Verification items for the finished model (mm, model axes). A direction names the side the tool comes from. Round coordinates to 2 decimals unless told otherwise and drop trailing zeros. Write each loop counter-clockwise with the first axis right and the second up, starting at its lowest first coordinate (ties: lowest second). Pieces come first, ordered by that corner, then holes. Notation, with made-up numbers: (-38.5, 1.25) - (-7.5, 1.25) arc R21 ccw to (-7.5, 5.25) - close; hole circle Ø6 at (27, 87). An arc over 180 degrees is marked (long way). Answer as a JSON object with one key per item and string values. Group by question number.
1) Mould release check, pull along Y, two halves, no side actions. Record for faces 5 (the cylindrical face through (-34.26, 7.31, 3.45)), 6 (the cylindrical face through (0, -15, 3)), 7 (the cylindrical face through (-14.287, -4.571, 3.451)), 8 (the cylindrical face through (39.73, 12.66, 3.45)): +Y half, -Y half, draft (parallel to the pull), parting line (faces both ways), or undercut.
2) Section check C-C (z = 6). Enter the section's corners in (x, y), then the cut area to 3 significant figures.
3) Section check B-B (y = -23.5). Enter the section's corners in (x, z), then the cut area to 3 significant figures.
4) Section check A-A (x = 0). Enter the section's corners in (y, z).
5) Go/stop test with flat-tipped pins: pin 1 Ø6 at (x, y) = (-7.5, -4.5) entering from +Z; pin 2 Ø1.5 at (x, z) = (-18, 6.5) entering from +Y; pin 3 Ø1 at (x, z) = (-6.5, 2.5) entering from +Y; pin 4 Ø2 at (y, z) = (18, 2) entering from +X. Record where each tip stops, or that it passes through.
6) Thickness scan on line 1 (Y direction, x = 17.5, z = 4.5); line 2 (X direction, y = -0.5, z = 6.5); line 3 (X direction, y = 17, z = 3). Record the ranges inside material, lowest first.
7) Set-up check for faces 1 (the flat face through (22.135, 2.461, 3.451)), 2 (the cylindrical face through (14.245, -4.7, 3.451)), 3 (the flat face through (-16.46, -15, 3.45)), 4 (the flat face through (19.6, 11.1, 3.5)): record each of +Z, -Z, +X, -X, +Y, -Y from which the full face is reachable in a straight line by a thin tool's end or side.
8) Section check D-D (y = 26). Enter the section's corners in (x, z).
```python
from build123d import *

# Parameters (mm, degrees)
F2_DEPTH = 7
F0_R     = 11.1
F3_DEPTH = 7.001
F4_R     = 3.652579
F5_DEPTH = 7.001


with BuildPart() as f2:
    # F1 (on Top) → F2 (new body)
    with BuildSketch(Plane.XY):
        with BuildLine():
            Line((-4.5, 29.528995), (-4.5, 14.309088))
            ThreePointArc((-4.5, 14.309088), (-8.816779, 12.135255), (-12.218175, 8.701506))
            Line((-12.218175, 8.701506), (-26.693166, 13.404716))
            ThreePointArc((-26.693166, 13.404716), (-39.661387, 12.886766), (-29.474319, 4.845207))
            Line((-29.474319, 4.845207), (-14.999328, 0.141997))
            ThreePointArc((-14.999328, 0.141997), (-14.265848, -4.635255), (-12.051247, -8.931262))
            Line((-12.051247, -8.931262), (-20.997284, -21.244425))
            ThreePointArc((-20.997284, -21.244425), (-24.512085, -33.737991), (-13.716131, -26.534492))
            Line((-13.716131, -26.534492), (-4.770094, -14.221329))
            ThreePointArc((-4.770094, -14.221329), (0, -15), (4.770094, -14.221329))
            Line((4.770094, -14.221329), (13.716131, -26.534492))
            ThreePointArc((13.716131, -26.534492), (24.512085, -33.737991), (20.997284, -21.244425))
            Line((20.997284, -21.244425), (12.051247, -8.931262))
            ThreePointArc((12.051247, -8.931262), (14.265848, -4.635255), (14.999328, 0.141997))
            Line((14.999328, 0.141997), (29.474319, 4.845207))
            ThreePointArc((29.474319, 4.845207), (39.661387, 12.886766), (26.693166, 13.404716))
            Line((26.693166, 13.404716), (12.218175, 8.701506))
            ThreePointArc((12.218175, 8.701506), (8.816779, 12.135255), (4.5, 14.309088))
            Line((4.5, 14.309088), (4.5, 29.528995))
            ThreePointArc((4.5, 29.528995), (0, 41.70245), (-4.5, 29.528995))
        make_face()
    extrude(amount=F2_DEPTH)

    # F0 (on Top) → F3 (cut, through all)
    with BuildSketch(Plane.XY):
        Circle(F0_R)
    extrude(amount=F3_DEPTH, mode=Mode.SUBTRACT)

    # F4 (on Top) → F5 (cut, through all)
    with BuildSketch(Plane.XY):
        with Locations((0, 35.191689)):
            Circle(F4_R)
        with Locations((-33.469285, 10.87483)):
            Circle(F4_R)
        with Locations((-20.685156, -28.470674)):
            Circle(F4_R)
        with Locations((20.685156, -28.470674)):
            Circle(F4_R)
        with Locations((33.469285, 10.87483)):
            Circle(F4_R)
    extrude(amount=F5_DEPTH, mode=Mode.SUBTRACT)


solid = f2.part
```
Returned:
{
 "1": {"face 5": "undercut", "face 6": "-Y half", "face 7": "undercut", "face 8": "parting line"},
 "2": {"outline": "(-29.47, 4.85) - (-15, 0.14) arc R15 ccw to (-12.05, -8.93) - (-21, -21.24) arc R6.92 ccw (long way) to (-13.72, -26.53) - (-4.77, -14.22) arc R15 ccw to (4.77, -14.22) - (13.72, -26.53) arc R6.92 ccw (long way) to (21, -21.24) - (12.05, -8.93) arc R15 ccw to (15, 0.14) - (29.47, 4.85) arc R6.92 ccw (long way) to (26.69, 13.4) - (12.22, 8.7) arc R15 ccw to (4.5, 14.31) - (4.5, 29.53) arc R6.92 ccw (long way) to (-4.5, 29.53) - (-4.5, 14.31) arc R15 ccw to (-12.22, 8.7) - (-26.69, 13.4) arc R6.92 ccw (long way) to start; hole circle Ø7.31 at (-33.47, 10.87); hole circle Ø7.31 at (-20.69, -28.47); hole circle Ø22.2 at (0, 0); hole circle Ø7.31 at (0, 35.19); hole circle Ø7.31 at (20.69, -28.47); hole circle Ø7.31 at (33.47, 10.87)", "area": "1,470 mm2"},
 "3": {"outline": "(-25.58, 0) - (-11.51, 0) - (-11.51, 7) - (-25.58, 7) - close; (11.51, 0) - (25.58, 0) - (25.58, 7) - (11.51, 7) - close", "area": "197 mm2"},
 "4": {"outline": "(-15, 0) - (-11.1, 0) - (-11.1, 7) - (-15, 7) - close; (11.1, 0) - (31.54, 0) - (31.54, 7) - (11.1, 7) - close; (38.84, 0) - (41.7, 0) - (41.7, 7) - (38.84, 7) - close"},
 "5": {"pin 1": "z = 7", "pin 2": "y = 10.82", "pin 3": "y = 38.23", "pin 4": "x = 36.05"},
 "6": {"line 1": "-34.4 to -30.26, -26.68 to -16.43, 0.95 to 10.42", "line 2": "-14.99 to -11.09, 11.09 to 14.99", "line 3": "-36.05 to -30.12, -4.5 to 4.5, 30.12 to 36.05"},
 "7": {"face 1": "+Z, -Z", "face 2": "+Z, -Z, +X", "face 3": "+Z, -Z, -X", "face 4": "+Z, -Z, +Y"},
 "8": {"outline": "(-4.5, 0) - (4.5, 0) - (4.5, 7) - (-4.5, 7) - close"}
}
